The model under review builds one solid part; all positions refer to its coordinate system, in mm. A direction names the side the tool comes from. Coordinates: 2 decimals unless noted, no trailing zeros. Loops run counter-clockwise (first coordinate to the right, second up) from the corner with the lowest first, then second, coordinate; pieces in that order, holes last. Notation, with made-up numbers: M 58,85 L 85,85 A22 cw 85,110 Z; hole C -6,19 d9. An arc over 180 degrees is marked long. One line per item, written item: value.
```python
from build123d import *

# Parameters (mm, degrees)
SKETCH1_W           = 25.654
SKETCH1_H           = 6.35
BOSS_EXTRUDE1_DEPTH = 101.6
FILLET1_R           = 0.508
FILLET2_R           = 1.016
SKETCH3_W           = 19.05
SKETCH3_H           = 63.5
BOSS_EXTRUDE3_DEPTH = 101.6
SKETCH4_R           = 6.3881
CUT_EXTRUDE1_DEPTH  = 25.4
FILLET3_R           = 2.54
FILLET4_R           = 1.27
FILLET5_R           = 1.27
CUT_EXTRUDE3_REACH  = 119.452
SKETCH5_R           = 3.2385
FILLET7_R           = 1.27
SKETCH6_W           = 0.127
SKETCH6_H           = 6.35
CUT_EXTRUDE4_DEPTH  = 114.192714866


with BuildPart() as part:
    # Sketch1 → Boss-Extrude1 (new body)
    with BuildSketch(Plane.XY):
        with Locations((0, 21.933756602)):
            Rectangle(SKETCH1_W, SKETCH1_H)
        Polygon((2.851307039, 16.218756602), (2.857235141, 18.758756602), (-2.856686021, 18.758756602), (-2.851856159, 16.218756602), (-7.55677456, 16.218756602), (-2.921, 10.757756602), (2.921, 10.757756602), (7.55622544, 16.218756602), align=None)
    extrude(amount=BOSS_EXTRUDE1_DEPTH)

    # Fillet1
    fillet1_edges = [part.edges().sort_by_distance(p)[0] for p in [
        (7.55622544, 16.218756602, 50.8),
        (-7.55677456, 16.218756602, 50.8),
    ]]
    fillet(fillet1_edges, radius=FILLET1_R)

    # Fillet2
    fillet2_edges = [part.edges().sort_by_distance(p)[0] for p in [
        (2.921, 10.757756602, 50.8),
        (-2.921, 10.757756602, 50.8),
    ]]
    fillet(fillet2_edges, radius=FILLET2_R)

    # Sketch3 → Boss-Extrude3 (add)
    with BuildSketch(Plane(origin=(0, 0, 0), x_dir=(-1, 0, 0), z_dir=(0, 0, -1))):
        with Locations((-22.352, -6.641243398)):
            Rectangle(SKETCH3_W, SKETCH3_H)
    extrude(amount=-BOSS_EXTRUDE3_DEPTH)

    # Sketch4 → Cut-Extrude1 (cut)
    with BuildSketch(Plane(origin=(31.877, 0, 0), x_dir=(0, 0, -1), z_dir=(1, 0, 0))):
        with Locations(Location((-19.177, -19.341243398, 0), (0, 0, 90))):
            Circle(SKETCH4_R)
        with Locations(Location((-82.423, -19.341243398, 0), (0, 0, 90))):
            Circle(SKETCH4_R)
    extrude(amount=-CUT_EXTRUDE1_DEPTH, mode=Mode.SUBTRACT)

    # Fillet3
    fillet3_edges = [part.edges().sort_by_distance(p)[0] for p in [
        (31.877, 25.108756602, 50.8),
    ]]
    fillet(fillet3_edges, radius=FILLET3_R)

    # Fillet4
    fillet4_edges = [part.edges().sort_by_distance(p)[0] for p in [
        (31.877, -25.729343398, 82.423),
        (31.877, -25.729343398, 19.177),
    ]]
    fillet(fillet4_edges, radius=FILLET4_R)

    # Fillet5
    fillet5_edges = [part.edges().sort_by_distance(p)[0] for p in [
        (8.255, 25.108756602, 0),
        (8.255, 25.108756602, 101.6),
        (12.827, -9.816243398, 0),
        (22.352, -38.391243398, 0),
        (31.877, -38.391243398, 50.8),
        (22.352, -38.391243398, 101.6),
        (12.827, -38.391243398, 50.8),
        (12.827, -9.816243398, 101.6),
        (31.877, -7.911243398, 0),
        (31.133051224, 24.364807826, 0),
        (31.877, -7.911243398, 101.6),
        (31.133051224, 24.364807826, 101.6),
    ]]
    fillet(fillet5_edges, radius=FILLET5_R)

    # Sketch5 → Cut-Extrude3 (cut, up to next)
    with BuildSketch(Plane(origin=(31.877, 0, 0), x_dir=(0, 0, -1), z_dir=(1, 0, 0)), mode=Mode.PRIVATE) as cut_extrude3_sk1:
        with Locations(Location((-82.423, 6.058756602, 0), (0, 0, 90))):
            Circle(SKETCH5_R)
    cut_extrude3_tool1 = extrude(cut_extrude3_sk1.sketch, amount=-CUT_EXTRUDE3_REACH, mode=Mode.PRIVATE) & part.part
    # Sketch5 → Cut-Extrude3 (cut, up to next)
    with BuildSketch(Plane(origin=(31.877, 0, 0), x_dir=(0, 0, -1), z_dir=(1, 0, 0)), mode=Mode.PRIVATE) as cut_extrude3_sk2:
        with Locations(Location((-19.177, 6.058756602, 0), (0, 0, 90))):
            Circle(SKETCH5_R)
    cut_extrude3_tool2 = extrude(cut_extrude3_sk2.sketch, amount=-CUT_EXTRUDE3_REACH, mode=Mode.PRIVATE) & part.part
    add(cut_extrude3_tool1.solids().sort_by_distance((31.877, 6.058757, 82.423))[0], mode=Mode.SUBTRACT)
    add(cut_extrude3_tool2.solids().sort_by_distance((31.877, 6.058757, 19.177))[0], mode=Mode.SUBTRACT)

    # Fillet7
    fillet7_edges = [part.edges().sort_by_distance(p)[0] for p in [
        (31.877, 2.820256602, 82.423),
        (31.877, 2.820256602, 19.177),
    ]]
    fillet(fillet7_edges, radius=FILLET7_R)

    # Sketch6 → Cut-Extrude4 (cut, through all)
    with BuildSketch(Plane.XY.offset(101.6)):
        with Locations((-12.7635, 21.933756602)):
            Rectangle(SKETCH6_W, SKETCH6_H)
    extrude(amount=-CUT_EXTRUDE4_DEPTH, mode=Mode.SUBTRACT)


solid = part.part
```
(1) Add section B-B on x = -8.5. State the section outline as (y, z) points.
Checks:
outline: M 18.76,0 L 23.84,0 A1.27 ccw 25.11,1.27 L 25.11,100.33 A1.27 ccw 23.84,101.6 L 18.76,101.6 Z
(2) Tool access review of faces 1 (the face through (-8, 18.759, 50)), 2 (the face through (21.841, -16.394, 76.756)), 3 (the face through (0, 10.758, 50)): name each direction out of +Z, -Z, +X, -X, +Y, -Y from which nothing blocks a thin tool from reaching the whole face with its end or side.
Checks:
face 1: +Z, -Z, -X
face 2: +X, -X
face 3: +Z, -Z, -X, -Y
(3) Add section A-A on y = -32.5. State the section outline as (x, z) points.
Checks:
outline: M 12.83,1.27 A1.27 ccw 14.1,0 L 30.61,0 A1.27 ccw 31.88,1.27 L 31.88,100.33 A1.27 ccw 30.61,101.6 L 14.1,101.6 A1.27 ccw 12.83,100.33 Z
(4) Draft analysis for pull direction Y (two halves, no side actions). For faces 4 (the face through (31.877, -8, 50)), 5 (the face through (5.01, 13.22, 50.09)), 6 (the face through (5, 16.219, 50)), state which applies: pulls with the +Y half, pulls with the -Y half, needs draft (parallel to the pull), parting line crosses it, or undercut.
Checks:
face 4: needs draft
face 5: pulls with the -Y half
face 6: undercut
(5) Add section C-C on z = 35. State the section outline as (x, y) points.
Checks:
outline: M -12.7,18.76 L -2.86,18.76 L -2.85,16.22 L -6.46,16.22 A0.51 ccw -6.85,15.38 L -3.23,11.12 A1.02 ccw -2.45,10.76 L 2.45,10.76 A1.02 ccw 3.23,11.12 L 6.85,15.38 A0.51 ccw 6.46,16.22 L 2.85,16.22 L 2.86,18.76 L 12.83,18.76 L 12.83,-37.12 A1.27 ccw 14.1,-38.39 L 30.61,-38.39 A1.27 ccw 31.88,-37.12 L 31.88,22.57 A2.54 ccw 29.34,25.11 L -12.7,25.11 Z
(6) To check wall thickness, follow L1, parallel to Z at x = 28, y = 6; L2, parallel to Z at x = 28, y = -17.5; L3, parallel to X at y = 5, z = 37. State the ranges of each line that lie inside material, in increasing order. Write a range as [from, to].
Checks:
L1: [0, 15.94], [22.41, 79.19], [85.66, 101.6]
L2: [0, 13.06], [25.29, 76.31], [88.54, 101.6]
L3: [12.83, 31.88]
(7) Insertion check: pin 1 Ø9 at (x, z) = (7.5, 60) entering from -Y; pin 2 Ø12 at (x, y) = (1, -25) entering from +Z; pin 3 Ø8.5 at (y, z) = (6.06, 19.18) entering from -X; pin 4 Ø14.5 at (y, z) = (-19.34, 19.18) entering from +X. Each pin has a flat end and moves straight along its axis. Give the tip position at first contact, or say it passes through.
Checks:
pin 1: y = 10.92
pin 2: through
pin 3: x = 12.83
pin 4: x = 31.81
(8) Add section D-D on y = 17.5. State the section outline as (x, z) points.
Checks:
outline: M -2.85,0 L 2.85,0 L 2.85,101.6 L -2.85,101.6 Z; M 12.83,1.27 A1.27 ccw 14.1,0 L 30.61,0 A1.27 ccw 31.88,1.27 L 31.88,100.33 A1.27 ccw 30.61,101.6 L 14.1,101.6 A1.27 ccw 12.83,100.33 Z
